```python
from build123d import *

# Parameters (mm, degrees)
F0_R     = 15
F1_DEPTH = 5
F2_R     = 2.5
F3_DEPTH = 25.4


with BuildPart() as f1:
    # F0 (on Front) → F1 (new body)
    with BuildSketch(Plane.XZ):
        Circle(F0_R)
    extrude(amount=F1_DEPTH)

    # F2 (on face) → F3 (join)
    with BuildSketch(Plane.XZ.offset(5)):
        with Locations((-6.495191, -3.75)):
            Circle(F2_R)
        with Locations((0, 7.5)):
            Circle(F2_R)
        with Locations((6.495191, -3.75)):
            Circle(F2_R)
    extrude(amount=F3_DEPTH)

    # F4 (on Right) → F5 (revolve, cut)
    with BuildSketch(Plane.YZ):
        Polygon((-20.142939, 0), (-30.415036, 10.272097), (-30.415036, 0), align=None)
    revolve(axis=Axis((0, -21.627579, 0), (0, -1, 0)), mode=Mode.SUBTRACT)


solid = f1.part
```
Part model, mm, in its own coordinate system. A direction names the side the tool comes from. Coordinates: 2 decimals unless noted, no trailing zeros. Order: outer loops, then holes, each group sorted by start corner. A loop starts at its lowest first (then second) coordinate and runs counter-clockwise, first axis right, second up. Notation, with made-up numbers: (-11.75, 67.5) - (9.25, 67.5) arc R28 cw to (9.25, 105.5) - close; hole circle Ø1 at (65.5, -18). An arc over 180 degrees is marked (long way). Return JSON: item names as keys, results as strings. Group by question number.
Item 1: Pin check, flat tips, straight feed: pin 1 (4 mm diameter, centred on y = -23.5, z = -4, fed in from +X); pin 2 (2 mm diameter, centred on x = 6.5, y = -26.5, fed in from +Z); pin 3 (1 mm diameter, centred on y = -22.5, z = -6, fed in from -X). Stop position of each tip, or through.
Item 2: Which spindle directions (+Z, -Z, +X, -X, +Y, -Y) get a long thin tool onto all of the face, cutting with end or side? Do faces 1 (the face through (0, -5, 0)), 2 (the face through (6.51, -27.68, -3.8)), 3 (the face through (-14.985, -2.465, 0.66)). Say none if no direction does.
Item 3: Cut at A-A (y = -20). List the corners of the cut face in (x, z), plus the area to 3 significant figures.
Item 4: Cut at B-B (x = 0). List the corners of the cut face in (y, z).
Item 5: Drill centre lines: probe 1 along Y at (x, z) = (3, -5.75); probe 2 along X at (y, z) = (-28, -2.75); probe 3 along Z at (x, y) = (6.5, -11). Where is each one in solid material? Low to high. Write a range as from..to.
Item 6: Cut at C-C (y = -4). List the corners of the cut face in (x, z).
Item 7: Pull direction X, two halves, no side cores. Call faces 4 (the face through (0, -17, 10)), 5 (the face through (0, 0, 0)), 6 (the face through (-6.543, -27.678, -3.736)): pulls with the +X half, pulls with the -X half, needs draft (parallel to the pull), parting line crosses it, or undercut.
Item 8: Cut at D-D (z = 0). List the corners of the cut face in (x, y).
Check values:
{
 "1": {"pin 1": "stops at x = 9", "pin 2": "stops at z = -1.25", "pin 3": "stops at x = -8.28"},
 "2": {"face 1": "-Y", "face 2": "+Z, -Y", "face 3": "+Y, -Y"},
 "3": {"outline": "circle Ø5 at (-6.5, -3.75); circle Ø5 at (0, 7.5); circle Ø5 at (6.5, -3.75)", "area": "58.9 mm2"},
 "4": {"outline": "(-30.14, 10) - (-25.14, 5) - (-5, 5) - (-5, -15) - (0, -15) - (0, 15) - (-5, 15) - (-5, 10) - close"},
 "5": {"probe 1": "y = -5..0", "probe 2": "x = -8.79..-7.36, 7.36..8.79", "probe 3": "z = -6.25..-1.25"},
 "6": {"outline": "circle Ø30 at (0, 0)"},
 "7": {"face 4": "parting line crosses it", "face 5": "needs draft", "face 6": "undercut"},
 "8": {"outline": "(-15, -5) - (15, -5) - (15, 0) - (-15, 0) - close"}
}
